Here's how the part is built. I have some questions about the finished solid (model axes, mm). A direction names the side the tool comes from. Give positions to 0.01 mm unless a question says otherwise; leave off trailing zeros. Write each loop counter-clockwise with the first axis right and the second up, starting at its lowest first coordinate (ties: lowest second). Pieces come first, ordered by that corner, then holes. Notation, with made-up numbers: (16, -33) -> (53, -33) arc R15 ccw to (53, -26) -> close; hole circle Ø7 at (57.25, 79). An arc over 180 degrees is marked (long way). Return JSON: item names as keys, results as strings.
from build123d import *

# Parameters (mm, degrees)
SKETCH_1_W      = 25
SKETCH_1_H      = 10
EXTRUDE_1_DEPTH = 20
EXTRUDE_2_DEPTH = 5
EXTRUDE_3_DEPTH = 10


with BuildPart() as part:
    # Sketch 1 → Extrude 1 (new body)
    with BuildSketch(Plane(origin=(0, 0, 0), x_dir=(1, 0, 0), z_dir=(0, 1, 0))):
        with Locations((12.5, 5)):
            Rectangle(SKETCH_1_W, SKETCH_1_H)
    extrude(amount=EXTRUDE_1_DEPTH)

    # Sketch 1_3 → Extrude 2 (add)
    with BuildSketch(Plane(origin=(0, 0, 0), x_dir=(1, 0, 0), z_dir=(0, 1, 0))):
        Polygon((30, -10), (30, 0), (25, 0), (0, 0), (0, -10), align=None)
    extrude(amount=EXTRUDE_2_DEPTH)

    # Sketch 2 → Extrude 3 (add)
    with BuildSketch(Plane(origin=(30, 0, 0), x_dir=(0, 0, -1), z_dir=(1, 0, 0))):
        Polygon((-5, 5), (0, 5), (0, 11.350931175), (0, 15), (-10, 15), (-10, 10), (-5, 10), align=None)
    extrude(amount=-EXTRUDE_3_DEPTH)


solid = part.part
1. Suppose I cut it at B-B, the plane x = 24.25. List the corners of the cut face in (y, z) for me, and give its area (3 significant figures).
Taken from the geometry:
{"outline": "(0, -10) -> (20, -10) -> (20, 0) -> (15, 0) -> (15, 10) -> (10, 10) -> (10, 5) -> (5, 5) -> (5, 10) -> (0, 10) -> close", "area": "325 mm²"}
2. Suppose I cut it at C-C, the plane z = 3.5. List the corners of the cut face in (x, y) for me.
Taken from the geometry:
{"outline": "(0, 0) -> (30, 0) -> (30, 15) -> (20, 15) -> (20, 5) -> (0, 5) -> close"}
3. Which directions (+Z, -Z, +X, -X, +Y, -Y) give clear straight access to the entire face, cutting with the end or side of a thin tool? Please do faces 4 (the face through (25, 10, 8)), 5 (the face through (20, 11, 4)), 6 (the face through (25, 10, -5)).
Taken from the geometry:
{"face 4": "+Z, +X, -X", "face 5": "+Z, -X, +Y", "face 6": "-Z, +X, +Y, -Y"}
4. For pin 1 Ø6 at (x, z) = (7, 4.5) entering from +Y; pin 2 Ø1 at (y, z) = (3.5, 1) entering from -X; pin 3 Ø8 at (y, z) = (13.5, -4.5) entering from +X; pin 4 Ø1.5 at (x, y) = (26.5, 8) entering from +Z, each with a flat end and sliding along its axis, tell me the tip position at first contact or that it passes through.
Taken from the geometry:
{"pin 1": "stops at y = 5", "pin 2": "stops at x = 0", "pin 3": "stops at x = 25", "pin 4": "stops at z = 5"}
5. Suppose I cut it at D-D, the plane x = 6.5. List the corners of the cut face in (y, z) for me.
Taken from the geometry:
{"outline": "(0, -10) -> (20, -10) -> (20, 0) -> (5, 0) -> (5, 10) -> (0, 10) -> close"}
6. If we mould it in two halves opening along Y, with no side actions, what happens to faces 1 (the face through (11, 5, 5)), 2 (the face through (15, 2, 10)), 3 (the face through (25, 15, 5))? For each: released by +Y, released by -Y, zero draft, split by the parting line, or undercut.
Taken from the geometry:
{"face 1": "undercut", "face 2": "zero draft", "face 3": "released by +Y"}
7. Suppose I cut it at A-A, the plane y = 13.25. List the corners of the cut face in (x, z) for me.
Taken from the geometry:
{"outline": "(0, -10) -> (25, -10) -> (25, 0) -> (30, 0) -> (30, 10) -> (20, 10) -> (20, 0) -> (0, 0) -> close"}
8. If I drill on line 1 (Y direction, x = 28.5, z = 8); line 2 (Y direction, x = 7, z = 3); line 3 (Z direction, x = 19.5, y = 9.75), over which ranges is the centre line in solid material (lowest first)? Write a range as [from, to].
Taken from the geometry:
{"line 1": "y = [0, 5], [10, 15]", "line 2": "y = [0, 5]", "line 3": "z = [-10, 0]"}
